Geometry: final body of the model. Coordinates: model frame, mm. A direction names the side the tool comes from. Give positions to 0.01 mm unless a question says otherwise; leave off trailing zeros. Write each loop counter-clockwise with the first axis right and the second up, starting at its lowest first coordinate (ties: lowest second). Pieces come first, ordered by that corner, then holes. Notation, with made-up numbers: M -16.5,-35.75 L 2.5,-35.75 A28 ccw 2.5,-17.75 Z; hole C -1,47 d1. An arc over 180 degrees is marked long. Answer as a JSON object with one key per item and string values.
from build123d import *

# Parameters (mm, degrees)
SKETCH1_R           = 7.93
SKETCH1_R_2         = 3.17
BOSS_EXTRUDE1_DEPTH = 7.42
SKETCH2_R           = 6.12
SKETCH2_R_2         = 3.17
BOSS_EXTRUDE2_DEPTH = 7.02
SKETCH3_R           = 7.93
SKETCH3_R_2         = 3.17
BOSS_EXTRUDE3_DEPTH = 1.5
SKETCH4_R           = 1.675
CUT_EXTRUDE1_DEPTH  = 8.93
CIRPATTERN1_COUNT   = 2
CIRPATTERN1_ANGLE   = 90


with BuildPart() as part:
    # Sketch1 → Boss-Extrude1 (new body)
    with BuildSketch(Plane(origin=(0, 0, 0), x_dir=(1, 0, 0), z_dir=(0, 1, 0))):
        Circle(SKETCH1_R)
        Circle(SKETCH1_R_2, mode=Mode.SUBTRACT)
    extrude(amount=BOSS_EXTRUDE1_DEPTH)

    # Sketch2 → Boss-Extrude2 (add)
    with BuildSketch(Plane(origin=(0, 7.42, 0), x_dir=(1, 0, 0), z_dir=(0, 1, 0))):
        Circle(SKETCH2_R)
        Circle(SKETCH2_R_2, mode=Mode.SUBTRACT)
    extrude(amount=BOSS_EXTRUDE2_DEPTH)

    # Sketch3 → Boss-Extrude3 (add)
    with BuildSketch(Plane(origin=(0, 14.44, 0), x_dir=(1, 0, 0), z_dir=(0, 1, 0))):
        Circle(SKETCH3_R)
        Circle(SKETCH3_R_2, mode=Mode.SUBTRACT)
    extrude(amount=BOSS_EXTRUDE3_DEPTH)

    # Sketch4 → Cut-Extrude1 (cut, through all)
    with BuildSketch(Plane(origin=(0, 0, 0), x_dir=(0, 0, -1), z_dir=(1, 0, 0))):
        with Locations((0, 3.71)):
            Circle(SKETCH4_R)
    cut_extrude1 = extrude(amount=-CUT_EXTRUDE1_DEPTH, mode=Mode.SUBTRACT)

    # CirPattern1: Cut-Extrude1 ×2 about axis
    cirpattern1_axis = Axis((0, 7.42, 0), (0, 1, 0))
    for i in range(1, CIRPATTERN1_COUNT):
        add(cut_extrude1.rotate(cirpattern1_axis, i * CIRPATTERN1_ANGLE / (CIRPATTERN1_COUNT - 1)), mode=Mode.SUBTRACT)


solid = part.part
1) Cut plane D-D on x = -6.5. Return loops of the section in (y, z) (3 decimals).
Geometry check:
{"outline": "M 0,-4.543 L 7.42,-4.543 L 7.42,4.543 L 0,4.543 Z; M 14.44,-4.543 L 15.94,-4.543 L 15.94,4.543 L 14.44,4.543 Z; hole C 3.71,0 d3.35"}
2) Cut plane C-C on y = 2.75. Return loops of the section in (x, z).
Geometry check:
{"outline": "M -7.81,-1.37 A7.93 ccw long 1.37,7.81 L 1.37,2.86 A3.17 cw long -2.86,-1.37 Z; M -7.81,1.37 L -2.86,1.37 A3.17 cw -1.37,2.86 L -1.37,7.81 A7.93 ccw Z"}
3) Cut plane A-A on z = 0. Return loops of the section in (x, y) (3 decimals), and give its area (3 significant figures).
Geometry check:
{"outline": "M -7.93,0 L -3.17,0 L -3.17,2.035 L -7.93,2.035 Z; M -7.93,5.385 L -3.17,5.385 L -3.17,15.94 L -7.93,15.94 L -7.93,14.44 L -6.12,14.44 L -6.12,7.42 L -7.93,7.42 Z; M 3.17,0 L 7.93,0 L 7.93,7.42 L 6.12,7.42 L 6.12,14.44 L 7.93,14.44 L 7.93,15.94 L 3.17,15.94 Z", "area": "110 mm2"}
4) Set-up query: faces 4 (the cylindrical face through (-6.29, 15.18, 4.83)), 5 (the cylindrical face through (1.673, 3.784, 5.276)), 6 (the cylindrical face through (-5.274, 3.784, 1.673)), 7 (the flat face through (4, 7.42, 5)), 8 (the flat face through (-0.1, 0, 3.4)). Return all of +Z, -Z, +X, -X, +Y, -Y with unobstructed straight access to the full face (end or side cutting, diameter ignored); none if empty.
Geometry check:
{"face 4": "+Y, -Y", "face 5": "+Z", "face 6": "-X", "face 7": "none", "face 8": "+Z, -Z, +X, -X, -Y"}
5) Line query: line 1 (Y direction, x = -6, z = 3.75); line 2 (Z direction, x = 0, y = 12). Output: solid intervals per line, ascending. Write a range as from..to.
Geometry check:
{"line 1": "y = 0..7.42, 14.44..15.94", "line 2": "z = -6.12..-3.17, 3.17..6.12"}
6) Cut plane B-B on x = 0. Return loops of the section in (y, z) (3 decimals).
Geometry check:
{"outline": "M 0,-7.93 L 7.42,-7.93 L 7.42,-6.12 L 14.44,-6.12 L 14.44,-7.93 L 15.94,-7.93 L 15.94,-3.17 L 0,-3.17 Z; M 0,3.17 L 2.035,3.17 L 2.035,7.93 L 0,7.93 Z; M 5.385,3.17 L 15.94,3.17 L 15.94,7.93 L 14.44,7.93 L 14.44,6.12 L 7.42,6.12 L 7.42,7.93 L 5.385,7.93 Z"}
7) Contact query for flat-ended pins moving along their axis: P1, Ø6, axis at y = 12, z = 2.5, coming from the -X side; P2, Ø1, axis at y = 12, z = -1.5, coming from the -X side; P3, Ø1.5, axis at x = -0.5, y = 8.5, coming from the +Z side; P4, Ø1.5, axis at x = -1, z = 0.5, coming from the +Y side. Output: stop coordinate, or through.
Geometry check:
{"P1": "stops at x = -7.89", "P2": "stops at x = -6.04", "P3": "stops at z = 6.12", "P4": "passes through"}
8) Pull-direction query (Z, two-part tool) for faces 1 (the cylindrical face through (-4.86, 10.88, 3.72)), 2 (the flat face through (4, 14.44, 5)), 3 (the cylindrical face through (1.704, 7.858, -2.673)); classes: pulls with the +Z half, pulls with the -Z half, needs draft (parallel to the pull), parting line crosses it, or undercut.
Geometry check:
{"face 1": "parting line crosses it", "face 2": "needs draft", "face 3": "undercut"}
